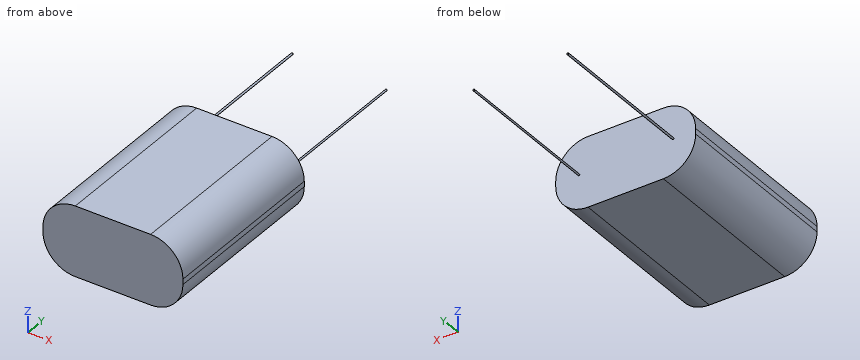
from build123d import *

# Parameters (mm, degrees)
SKETCH1_W           = 16.51
SKETCH1_H           = 20.955
BOSS_EXTRUDE1_DEPTH = 8.255
FILLET1_R           = 3.81
SKETCH2_R           = 0.095779186
SKETCH2_R_2         = 0.11203659
BOSS_EXTRUDE2_DEPTH = 18.161


with BuildPart() as part:
    # Sketch1 → Boss-Extrude1 (new body)
    with BuildSketch(Plane.XY):
        with Locations((-5.510011418, -21.415196798)):
            Rectangle(SKETCH1_W, SKETCH1_H)
    extrude(amount=BOSS_EXTRUDE1_DEPTH)

    # Fillet1
    fillet1_edges = [part.edges().sort_by_distance(p)[0] for p in [
        (-13.765011418, -21.415196798, 8.255),
        (2.744988582, -21.415196798, 8.255),
        (-13.765011418, -21.415196798, 0),
        (2.744988582, -21.415196798, 0),
    ]]
    fillet(fillet1_edges, radius=FILLET1_R)

    # Sketch2 → Boss-Extrude2 (add)
    with BuildSketch(Plane(origin=(0, -10.937696798, 0), x_dir=(1, 0, 0), z_dir=(0, 1, 0))):
        with Locations(Location((0, -4.160603471, 0), (0, 0, 90))):  # turned: the seam where the file's is
            Circle(SKETCH2_R)
        with Locations(Location((-11.093960289, -4.256382657, 0), (0, 0, 90))):  # turned: the seam where the file's is
            Circle(SKETCH2_R_2)
    extrude(amount=BOSS_EXTRUDE2_DEPTH)


solid = part.part
Work out the finished part from the listing and answer in its coordinate system (mm). Round coordinates to 2 decimals unless told otherwise and drop trailing zeros. Write each loop counter-clockwise with the first axis right and the second up, starting at its lowest first coordinate (ties: lowest second). Pieces come first, ordered by that corner, then holes.
1) A cutting plane is placed at B-B (x = -1.75). Give the vertices of the cut face in (y, z) (3 decimals).
2) Given pin 1 Ø4 at (x, z) = (-7.5, 4.5) entering from +Y; pin 2 Ø5 at (x, y) = (-2.5, -1) entering from +Z, each flat-ended and moving along its own axis, determine where each tip first touches the part or whether it passes through.
3) A cutting plane is placed at A-A (y = -11.5). Give the vertices of the cut face in (x, z) (3 decimals), plus the area to 3 significant figures.
4) A cutting plane is placed at D-D (y = -3). Give the vertices of the cut face in (x, z), plus the area to 3 significant figures.
5) Straight lines are drawn through the part: line 1 (Y direction, x = -13, z = 1.75); line 2 (X direction, y = -12, z = 7.75); line 3 (X direction, y = -25, z = 7). For each, find the intervals that lie inside material, in ascending order.
6) A cutting plane is placed at C-C (z = 5.25). Give the vertices of the cut face in (x, y).
Completed:
1. outline: (-31.893, 0) - (-10.938, 0) - (-10.938, 8.255) - (-31.893, 8.255) - close
2. pin 1: stops at y = -10.94
2. pin 2: stops at z = 4.26
3. outline: (-13.765, 3.81) arc R3.81 ccw to (-9.955, 0) - (-1.065, 0) arc R3.81 ccw to (2.745, 3.81) - (2.745, 4.445) arc R3.81 ccw to (-1.065, 8.255) - (-9.955, 8.255) arc R3.81 ccw to (-13.765, 4.445) - close
3. area: 124 mm2
4. outline: circle Ø0.22 at (-11.09, 4.26); circle Ø0.19 at (0, 4.16)
4. area: 0.0683 mm2
5. line 1: y = -31.89 to -10.94
5. line 2: x = -11.85 to 0.83
5. line 3: x = -12.78 to 1.76
6. outline: (-13.68, -31.89) - (2.66, -31.89) - (2.66, -10.94) - (-13.68, -10.94) - close
